Geometry: final body of the model. Coordinates: model frame, mm. Give positions to 0.01 mm unless a question says otherwise; leave off trailing zeros. Order: outer loops, then holes, each group sorted by start corner. A loop starts at its lowest first (then second) coordinate and runs counter-clockwise, first axis right, second up. Notation, with made-up numbers: (-8, -7) - (-4, -7) arc R14 cw to (-4, 14) - close; hole circle Ø10 at (54.25, -17). An arc over 180 degrees is marked (long way). One line per item, written item: value.
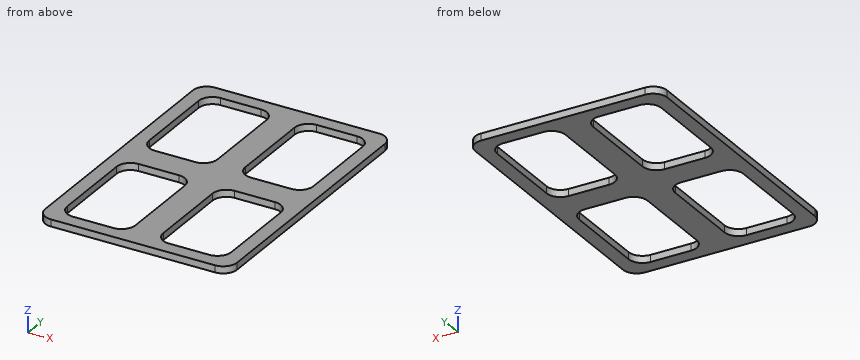
```python
from build123d import *

# Parameters (mm, degrees)
SKETCH_1_W          = 138
SKETCH_1_H          = 200
EXTRUDE_1_DEPTH     = 5
SKETCH_2_W          = 49
SKETCH_2_H          = 80
CUT_EXTRUDE_2_DEPTH = 5
FILLET_1_R          = 10


with BuildPart() as part:
    # 草图1 → 凸台-拉伸1 (new body)
    with BuildSketch(Plane.XY):
        Rectangle(SKETCH_1_W, SKETCH_1_H)
    extrude(amount=EXTRUDE_1_DEPTH)

    # 草图2 → 切除-拉伸2 (cut)
    with BuildSketch(Plane.XY.offset(5)):
        with Locations((34.5, 50)):
            Rectangle(SKETCH_2_W, SKETCH_2_H)
        with Locations((-34.5, 50)):
            Rectangle(SKETCH_2_W, SKETCH_2_H)
        with Locations((34.5, -50)):
            Rectangle(SKETCH_2_W, SKETCH_2_H)
        with Locations((-34.5, -50)):
            Rectangle(SKETCH_2_W, SKETCH_2_H)
    extrude(amount=-CUT_EXTRUDE_2_DEPTH, mode=Mode.SUBTRACT)

    # 圆角1
    fillet_1_edges = [part.edges().sort_by_distance(p)[0] for p in [
        (-10, 90, 2.5),
        (-10, 10, 2.5),
        (-59, 10, 2.5),
        (-59, 90, 2.5),
        (10, -90, 2.5),
        (10, -10, 2.5),
        (59, -10, 2.5),
        (59, -90, 2.5),
        (-10, -90, 2.5),
        (-59, -90, 2.5),
        (-59, -10, 2.5),
        (-10, -10, 2.5),
        (10, 10, 2.5),
        (10, 90, 2.5),
        (59, 90, 2.5),
        (59, 10, 2.5),
        (-69, 100, 2.5),
        (69, 100, 2.5),
        (69, -100, 2.5),
        (-69, -100, 2.5),
    ]]
    fillet(fillet_1_edges, radius=FILLET_1_R)


solid = part.part
```
1) Material intervals for line 1 along X through (y, z) = (-80, 3.3); line 2 along Y through (x, z) = (-40, 3.2); line 3 along Y through (x, z) = (-17, 1.8), sorted ascending.
Answers below:
line 1: -69 to -59, -10 to 10, 59 to 69
line 2: -100 to -90, -10 to 10, 90 to 100
line 3: -100 to -89.54, -10.46 to 10.46, 89.54 to 100
2) Section A-A, the plane x = -24. Return loops of the section in (y, z).
Answers below:
outline: (-100, 0) - (-90, 0) - (-90, 5) - (-100, 5) - close; (-10, 0) - (10, 0) - (10, 5) - (-10, 5) - close; (90, 0) - (100, 0) - (100, 5) - (90, 5) - close
3) Section C-C, the plane z = 2.9. Count the separate pieces of the cut face and the enclosed holes in it, then the cut area to 3 significant figures.
Answers below:
separate pieces: 1
enclosed holes: 4
area: 12,200 mm^2
4) Section B-B, the plane y = -52. Return loops of the section in (x, z).
Answers below:
outline: (-69, 0) - (-59, 0) - (-59, 5) - (-69, 5) - close; (-10, 0) - (10, 0) - (10, 5) - (-10, 5) - close; (59, 0) - (69, 0) - (69, 5) - (59, 5) - close
